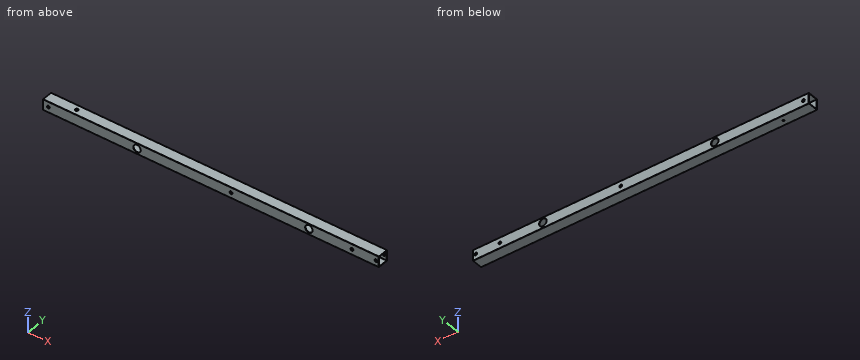
Autodesk Inventor part; units mm, degrees
ref_plane "YZ Plane" through (0, 0, 0) normal (1, 0, 0) x (0, 1, 0)
ref_plane "XZ Plane" through (0, 0, 0) normal (0, 1, 0) x (-1, 0, 0)
ref_plane "XY Plane" through (0, 0, 0) normal (0, 0, 1) x (1, 0, 0)
sketch "Skizze1" plane through (0, 0, 0) normal (1, 0, 0) x (0, 1, 0)
  line L0 (-19, 20) -> (19, 20)
  line L1 (20, 19) -> (20, -19)
  line L2 (19, -20) -> (-19, -20)
  line L3 (-20, -19) -> (-20, 19)
  line L4 (-20, 20) -> (20, -20) construction
  line L5 (20, 20) -> (-20, -20) construction
  line L6 (-17.5, 18) -> (17.5, 18)
  line L7 (18, 17.5) -> (18, -17.5)
  line L8 (17.5, -18) -> (-17.5, -18)
  line L9 (-18, -17.5) -> (-18, 17.5)
  line L10 (-18, 18) -> (18, -18) construction
  line L11 (18, 18) -> (-18, -18) construction
  arc A0 (20, 19) -> (19, 20) centre (19, 19) ccw
  arc A1 (-19, 20) -> (-20, 19) centre (-19, 19) ccw
  arc A2 (-20, -19) -> (-19, -20) centre (-19, -19) ccw
  arc A3 (19, -20) -> (20, -19) centre (19, -19) ccw
  arc A4 (18, 17.5) -> (17.5, 18) centre (17.5, 17.5) ccw
  arc A5 (-17.5, 18) -> (-18, 17.5) centre (-17.5, 17.5) ccw
  arc A6 (17.5, -18) -> (18, -17.5) centre (17.5, -17.5) ccw
  arc A7 (-18, -17.5) -> (-17.5, -18) centre (-17.5, -17.5) ccw
  point P0 (0, 0)
  dimension "d0" = 40
  dimension "d1" = 40
  dimension "d2" = 36
  dimension "d3" = 36
  dimension "d4" = 1
  dimension "d5" = 0.5
extrude "Extrusion1" add sketch "Skizze1" along normal blind 1250
sketch "Skizze2" plane through (0, 20, 19) normal (0, 1, 0) x (1, 0, 0)
  line L0 (0, 19) -> (20, 19)
  line L1 (1250, 38) -> (1250, 0)
  line L2 (1250, 19) -> (1150, 19)
  circle A0 centre (1150, 19) radius 5.25
  circle A1 centre (20, 19) radius 5.25
  dimension "d9" = 20
  dimension "d10" = 100
  dimension "d11" = 10.5
  dimension "d12" = 10.5
extrude "Extrusion2" cut sketch "Skizze2" against normal blind 1250
sketch "Skizze3" plane through (0, -19, 20) normal (0, 0, 1) x (1, 0, 0)
  line L0 (0, 19) -> (110, 19)
  line L1 (1250, 0) -> (1250, 38)
  line L2 (1250, 19) -> (1240, 19)
  circle A0 centre (110, 19) radius 3.2
  dimension "d15" = 110
  dimension "d18" = 6.4
extrude "Extrusion3" cut sketch "Skizze3" against normal blind 1250
sketch "Skizze4" plane through (0, -19, 20) normal (0, 0, 1) x (1, 0, 0)
  line L0 (0, 19) -> (110, 19)
  circle A0 centre (110, 19) radius 5.5
  dimension "d21" = 110
  dimension "d22" = 11
extrude "Extrusion4" cut sketch "Skizze4" against normal blind 2
sketch "Skizze6" plane through (0, -20, -19) normal (0, -1, 0) x (1, 0, 0)
  circle A0 centre (1150, 19) radius 5.25
  line L0 (1150, 19) -> (350, 19)
  circle A1 centre (350, 19) radius 14
  point P0 (0, 19)
  dimension "d31" = 800
  dimension "d32" = 28
extrude "Extrusion6" cut sketch "Skizze6" against normal blind 40 contours A1
sketch "Skizze7" plane through (0, 20, 19) normal (0, 1, 0) x (1, 0, 0)
  line L0 (1250, 38) -> (1250, 0)
  line L1 (1250, 19) -> (1240, 19)
  circle A0 centre (1240, 19) radius 5.25
  point P0 (0, 19)
  dimension "d35" = 10
  dimension "d36" = 10.5
extrude "Extrusion7" cut sketch "Skizze7" against normal through all
sketch "Skizze8" plane through (0, -20, -19) normal (0, -1, 0) x (1, 0, 0)
  line L0 (1250, 1.5) -> (1250, 1)
  line L1 (1250, 1) -> (990.0005, 1.5)
  line L2 (0, 1.5) -> (1250, 1.5)
  line L3 (990.0005, 1.5) -> (970.0005, 1.5)
  line L4 (0, 0) -> (1250, 0)
  line L5 (990.0005, 0) -> (970.0005, 0)
  line L6 (990.0005, 0) -> (990.0005, 20)
  circle A0 centre (990.0005, 20) radius 14
  point P0 (0, 19)
  dimension "d39" = 260
  dimension "d40" = 20
  dimension "d41" = 20
  dimension "d42" = 20
  dimension "d43" = 28
extrude "Extrusion8" cut sketch "Skizze8" against normal through all contours A0
sketch "Skizze9" plane through (0, -20, -19) normal (0, -1, 0) x (1, 0, 0)
  line L0 (1250, 1.5) -> (1250, 36.5)
  line L1 (1250, 19) -> (700, 19)
  circle A0 centre (700, 19) radius 5.25
  point P0 (0, 19)
  dimension "d46" = 550
  dimension "d47" = 10.5
extrude "Extrusion9" cut sketch "Skizze9" against normal through all
properties part number "Längs_Traverse_vorne" material "Aluminium 6061"
Geometry check sheet. Reference: the model listing, model coordinates, mm. Coordinates: 2 decimals unless noted, no trailing zeros. Order: outer loops, then holes, each group sorted by start corner. A loop starts at its lowest first (then second) coordinate and runs counter-clockwise, first axis right, second up.
Item 1: Section check A-A (x = 350). Enter the section's corners in (y, z), plus the area to 3 significant figures.
Item 2: Section check B-B (x = 479). Enter the section's corners in (y, z), plus the area to 3 significant figures.
Item 3: Scan lines: line 1 along Y through (x, z) = (356, 14); line 2 along Z through (x, y) = (700, -19.45). Record each from-to range of solid material in increasing order.
Check sheet entries:
1. outline: (-20, -19) arc R1 ccw to (-19, -20) - (19, -20) arc R1 ccw to (20, -19) - (20, -14) - (18, -14) - (18, -17.5) arc R0.5 cw to (17.5, -18) - (-17.5, -18) arc R0.5 cw to (-18, -17.5) - (-18, -14) - (-20, -14) - close; (-20, 14) - (-18, 14) - (-18, 17.5) arc R0.5 cw to (-17.5, 18) - (17.5, 18) arc R0.5 cw to (18, 17.5) - (18, 14) - (20, 14) - (20, 19) arc R1 ccw to (19, 20) - (-19, 20) arc R1 ccw to (-20, 19) - close
1. area: 191 mm2
2. outline: (-20, -19) arc R1 ccw to (-19, -20) - (19, -20) arc R1 ccw to (20, -19) - (20, 19) arc R1 ccw to (19, 20) - (-19, 20) arc R1 ccw to (-20, 19) - close; hole (-18, -17.5) arc R0.5 ccw to (-17.5, -18) - (17.5, -18) arc R0.5 ccw to (18, -17.5) - (18, 17.5) arc R0.5 ccw to (17.5, 18) - (-17.5, 18) arc R0.5 ccw to (-18, 17.5) - close
2. area: 303 mm2
3. line 1: y = -20 to -18, 18 to 20
3. line 2: z = -19.89 to -5.25, 5.25 to 19.89
